Study the drawing (mm; zero at the part's minimum x, y, z) and answer. Coordinates: 2 decimals unless noted, no trailing zeros. Order: outer loops, then holes, each group sorted by start corner. A loop starts at its lowest first (then second) coordinate and runs counter-clockwise, first axis right, second up. Notation, with made-up numbers: (49, 71) -> (81, 71) arc R19 cw to (81, 90) -> close; hole circle Ø2 at (86, -3). An arc over 180 degrees is marked (long way). Write each question's results on one line, items separated by ' | '. Start each with the question number.
(1) Given pin 1 (3.5 mm diameter, centred on x = 11.43, y = 2.54, fed in from +Z); pin 2 (1 mm diameter, centred on x = 17.5, z = 15.5, fed in from -Y); pin 3 (4 mm diameter, centred on y = 19.5, z = 14, fed in from +X) (1 decimal); pin 4 (1 mm diameter, centred on x = 13.5, z = 11.5, fed in from -Y), each flat-ended and moving along its own axis, determine where each tip first touches the part or whether it passes through.
(2) Straight lines are drawn through the part: L1, parallel to Y at x = 11.43, z = 12.25; L2, parallel to X at y = 9.5, z = 1.25 (1 decimal); L3, parallel to X at y = 2.54, z = 4.75 (1 decimal). For each, find the intervals that lie inside material, in ascending order.
(3) The part is cut by section D-D, the plane z = 9. Give the vertices of the cut face in (x, y).
(4) The part is cut by section A-A, the plane x = 11.43. Give the vertices of the cut face in (y, z).
(5) Determine the mould class of the marked faces 1, 2, 3 and 4 for opening direction Y: +Y half, -Y half, draft (parallel to the pull), parting line (faces both ways), or undercut.
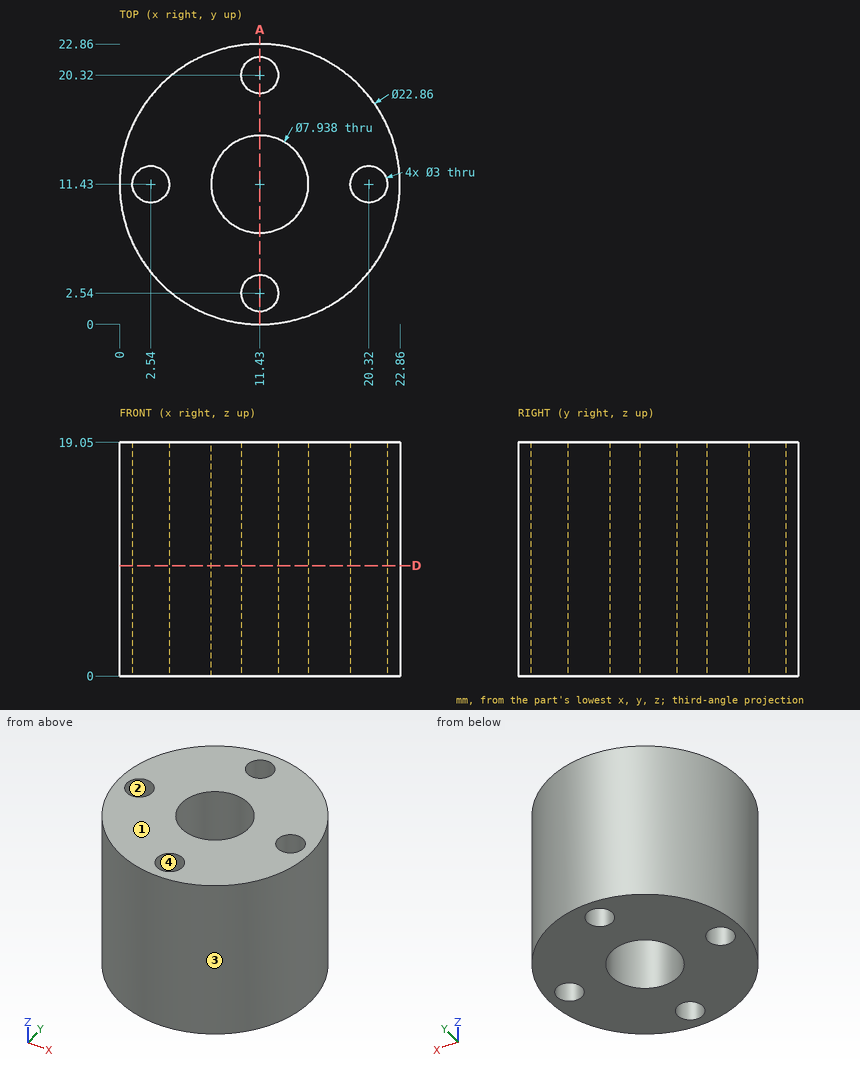
Established:
1) pin 1: stops at z = 19.05 | pin 2: stops at y = 1.45 | pin 3: stops at x = 21.1 | pin 4: stops at y = 0.11
2) L1: y = 0 to 1.04, 4.04 to 7.46, 15.4 to 18.82, 21.82 to 22.86 | L2: x = 0.2 to 8, 14.9 to 22.7 | L3: x = 4.2 to 9.9, 12.9 to 18.6
3) outline: circle Ø22.86 at (11.43, 11.43); hole circle Ø3 at (2.54, 11.43); hole circle Ø7.94 at (11.43, 11.43); hole circle Ø3 at (11.43, 2.54); hole circle Ø3 at (11.43, 20.32); hole circle Ø3 at (20.32, 11.43)
4) outline: (0, 0) -> (1.04, 0) -> (1.04, 19.05) -> (0, 19.05) -> close; (4.04, 0) -> (7.46, 0) -> (7.46, 19.05) -> (4.04, 19.05) -> close; (15.4, 0) -> (18.82, 0) -> (18.82, 19.05) -> (15.4, 19.05) -> close; (21.82, 0) -> (22.86, 0) -> (22.86, 19.05) -> (21.82, 19.05) -> close
5) face 1: draft | face 2: undercut | face 3: parting line | face 4: undercut
